from build123d import *

# Parameters (mm, degrees)
F0_W     = 73.9
F0_H     = 89.9
F0_W_2   = 69.9
F0_H_2   = 85.9
F1_DEPTH = 3
F2_DEPTH = 7
F3_DEPTH = 7


with BuildPart() as f1:
    # F0 (on Top) → F1 (new body)
    with BuildSketch(Plane.XY):
        with BuildLine():
            Line((40.45, -43.45), (40.45, 43.45))
            ThreePointArc((40.45, 43.45), (38.9855339059, 46.9855339059), (35.45, 48.45))
            Line((35.45, 48.45), (-35.45, 48.45))
            ThreePointArc((-35.45, 48.45), (-38.9855339059, 46.9855339059), (-40.45, 43.45))
            Line((-40.45, 43.45), (-40.45, -43.45))
            ThreePointArc((-40.45, -43.45), (-38.9855339059, -46.9855339059), (-35.45, -48.45))
            Line((-35.45, -48.45), (35.45, -48.45))
            ThreePointArc((35.45, -48.45), (38.9855339059, -46.9855339059), (40.45, -43.45))
        make_face()
        with BuildLine():
            ThreePointArc((-39.45, 43.45), (-38.2784271247, 46.2784271247), (-35.45, 47.45))
            Line((-35.45, 47.45), (35.45, 47.45))
            ThreePointArc((35.45, 47.45), (38.2784271247, 46.2784271247), (39.45, 43.45))
            Line((39.45, 43.45), (39.45, -43.45))
            ThreePointArc((39.45, -43.45), (38.2784271247, -46.2784271247), (35.45, -47.45))
            Line((35.45, -47.45), (-35.45, -47.45))
            ThreePointArc((-35.45, -47.45), (-38.2784271247, -46.2784271247), (-39.45, -43.45))
            Line((-39.45, -43.45), (-39.45, 43.45))
        make_face(mode=Mode.SUBTRACT)
        with BuildLine():
            Line((35.45, 47.45), (-35.45, 47.45))
            ThreePointArc((-35.45, 47.45), (-38.2784271247, 46.2784271247), (-39.45, 43.45))
            Line((-39.45, 43.45), (-39.45, -43.45))
            ThreePointArc((-39.45, -43.45), (-38.2784271247, -46.2784271247), (-35.45, -47.45))
            Line((-35.45, -47.45), (35.45, -47.45))
            ThreePointArc((35.45, -47.45), (38.2784271247, -46.2784271247), (39.45, -43.45))
            Line((39.45, -43.45), (39.45, 43.45))
            ThreePointArc((39.45, 43.45), (38.2784271247, 46.2784271247), (35.45, 47.45))
        make_face()
        Rectangle(F0_W, F0_H, mode=Mode.SUBTRACT)
        Rectangle(F0_W, F0_H)
        Rectangle(F0_W_2, F0_H_2, mode=Mode.SUBTRACT)
        Rectangle(F0_W_2, F0_H_2)
    extrude(amount=F1_DEPTH)

    # F0 (on Top) → F2 (join)
    with BuildSketch(Plane.XY):
        with BuildLine():
            Line((40.45, -43.45), (40.45, 43.45))
            ThreePointArc((40.45, 43.45), (38.9855339059, 46.9855339059), (35.45, 48.45))
            Line((35.45, 48.45), (-35.45, 48.45))
            ThreePointArc((-35.45, 48.45), (-38.9855339059, 46.9855339059), (-40.45, 43.45))
            Line((-40.45, 43.45), (-40.45, -43.45))
            ThreePointArc((-40.45, -43.45), (-38.9855339059, -46.9855339059), (-35.45, -48.45))
            Line((-35.45, -48.45), (35.45, -48.45))
            ThreePointArc((35.45, -48.45), (38.9855339059, -46.9855339059), (40.45, -43.45))
        make_face()
        with BuildLine():
            ThreePointArc((-39.45, 43.45), (-38.2784271247, 46.2784271247), (-35.45, 47.45))
            Line((-35.45, 47.45), (35.45, 47.45))
            ThreePointArc((35.45, 47.45), (38.2784271247, 46.2784271247), (39.45, 43.45))
            Line((39.45, 43.45), (39.45, -43.45))
            ThreePointArc((39.45, -43.45), (38.2784271247, -46.2784271247), (35.45, -47.45))
            Line((35.45, -47.45), (-35.45, -47.45))
            ThreePointArc((-35.45, -47.45), (-38.2784271247, -46.2784271247), (-39.45, -43.45))
            Line((-39.45, -43.45), (-39.45, 43.45))
        make_face(mode=Mode.SUBTRACT)
    extrude(amount=F2_DEPTH)

    # F0 (on Top) → F3 (join)
    with BuildSketch(Plane.XY):
        Rectangle(F0_W, F0_H)
        Rectangle(F0_W_2, F0_H_2, mode=Mode.SUBTRACT)
    extrude(amount=F3_DEPTH)


solid = f1.part
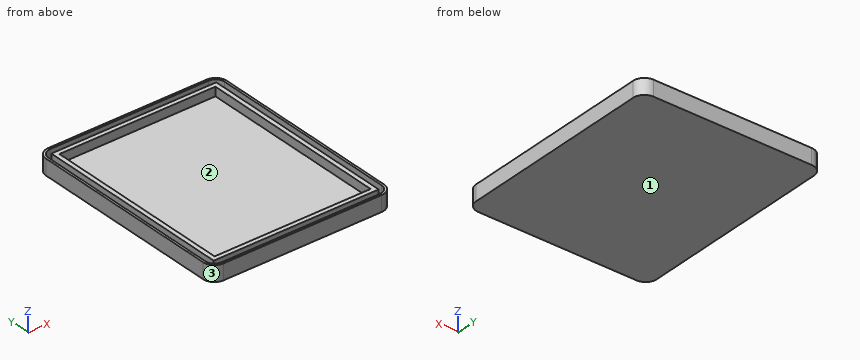
Geometry check sheet. Reference: the model listing, model coordinates, mm. Face numbers are marked on the shaded views. Give positions to 0.01 mm unless a question says otherwise; leave off trailing zeros. Loops run counter-clockwise (first coordinate to the right, second up) from the corner with the lowest first, then second, coordinate; pieces in that order, holes last. Notation, with made-up numbers: M 20.5,-12 L 25.5,-12 A7 cw 25.5,-4 Z; hole C 80,-6 d11. An arc over 180 degrees is marked long. Answer as a JSON object with one key per item and string values. Group by question number.
Item 1: Sectioned sample at B-B on y = 28. Record the boundary of the cut face in (x, z).
Item 2: Sectioned sample at C-C on x = 23.5. Record the boundary of the cut face in (y, z), plus the area to 3 significant figures.
Item 3: Material ranges on L1, parallel to Y at x = -5.5, z = 3.5; L2, parallel to X at y = -23.5, z = 6.75; L3, parallel to Y at x = -36.5, z = 5.5, recorded low to high.
Item 4: Mould release check, pull along X, two halves, no side actions. Record for the marked faces 1, 2 and 3: pulls with the +X half, pulls with the -X half, needs draft (parallel to the pull), parting line crosses it, or undercut.
Item 5: Sectioned sample at A-A on z = 5.5. Record the boundary of the cut face in (x, y), plus the area to 3 significant figures.
Findings below:
{
 "1": {"outline": "M -40.45,0 L 40.45,0 L 40.45,7 L 39.45,7 L 39.45,3 L 36.95,3 L 36.95,7 L 34.95,7 L 34.95,3 L -34.95,3 L -34.95,7 L -36.95,7 L -36.95,3 L -39.45,3 L -39.45,7 L -40.45,7 Z"},
 "2": {"outline": "M -48.45,0 L 48.45,0 L 48.45,7 L 47.45,7 L 47.45,3 L 44.95,3 L 44.95,7 L 42.95,7 L 42.95,3 L -42.95,3 L -42.95,7 L -44.95,7 L -44.95,3 L -47.45,3 L -47.45,7 L -48.45,7 Z", "area": "315 mm2"},
 "3": {"L1": "-48.45 to -47.45, -44.95 to -42.95, 42.95 to 44.95, 47.45 to 48.45", "L2": "-40.45 to -39.45, -36.95 to -34.95, 34.95 to 36.95, 39.45 to 40.45", "L3": "-48.34 to -47.31, -44.95 to 44.95, 47.31 to 48.34"},
 "4": {"face 1": "needs draft", "face 2": "undercut", "face 3": "pulls with the -X half"},
 "5": {"outline": "M -40.45,-43.45 A5 ccw -35.45,-48.45 L 35.45,-48.45 A5 ccw 40.45,-43.45 L 40.45,43.45 A5 ccw 35.45,48.45 L -35.45,48.45 A5 ccw -40.45,43.45 Z; M -36.95,-44.95 L 36.95,-44.95 L 36.95,44.95 L -36.95,44.95 Z; hole M -39.45,-43.45 A4 ccw -35.45,-47.45 L 35.45,-47.45 A4 ccw 39.45,-43.45 L 39.45,43.45 A4 ccw 35.45,47.45 L -35.45,47.45 A4 ccw -39.45,43.45 Z; hole M -34.95,-42.95 L 34.95,-42.95 L 34.95,42.95 L -34.95,42.95 Z", "area": "983 mm2"}
}
